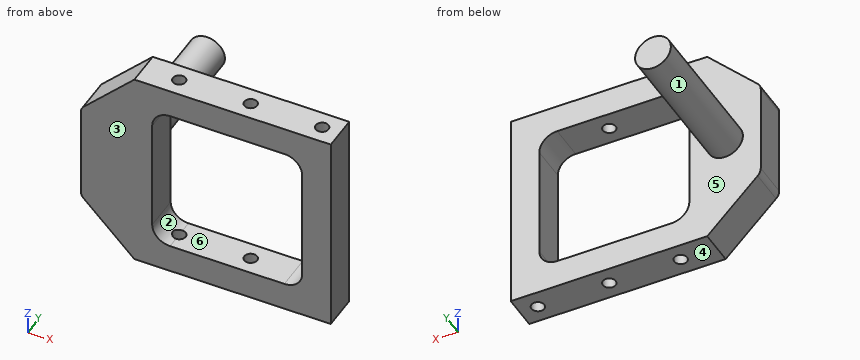
from build123d import *

# Parameters (mm, degrees)
SKETCH1_W          = 70
SKETCH1_H          = 10
EXTRUDE1_DEPTH     = 58
SKETCH2_R          = 5
EXTRUDE2_DEPTH     = 49
CUT_EXTRUDE1_DEPTH = 30
CHAMFER1_SIZE      = 15
FILLET1_R          = 3
SKETCH4_R          = 1.8
CUT_EXTRUDE2_DEPTH = 60


with BuildPart() as part:
    # Sketch1 → Extrude1 (new body)
    with BuildSketch(Plane.XY):
        with Locations((-10.032216865, -100)):
            Rectangle(SKETCH1_W, SKETCH1_H)
    extrude(amount=EXTRUDE1_DEPTH)

    # Sketch2 → Extrude2 (add)
    with BuildSketch(Plane.XZ.offset(105)):
        with Locations((-35.032216865, 28.7)):
            Circle(SKETCH2_R)
    extrude(amount=-EXTRUDE2_DEPTH)

    # Sketch3 → Cut-Extrude1 (cut)
    with BuildSketch(Plane.XZ.offset(105)):
        with BuildLine():
            Line((-20.032216865, 50), (11.967783135, 50))
            ThreePointArc((11.967783135, 50), (15.503317041, 48.535533906), (16.967783135, 45))
            Line((16.967783135, 45), (16.967783135, 13))
            ThreePointArc((16.967783135, 13), (15.503317041, 9.464466094), (11.967783135, 8))
            Line((11.967783135, 8), (-20.032216865, 8))
            ThreePointArc((-20.032216865, 8), (-23.567750771, 9.464466094), (-25.032216865, 13))
            Line((-25.032216865, 13), (-25.032216865, 45))
            ThreePointArc((-25.032216865, 45), (-23.567750771, 48.535533906), (-20.032216865, 50))
        make_face()
    extrude(amount=-CUT_EXTRUDE1_DEPTH, mode=Mode.SUBTRACT)

    # Chamfer1
    chamfer1_edges = [part.edges().sort_by_distance(p)[0] for p in [
        (-45.032216865, -100, 58),
        (-45.032216865, -100, 0),
    ]]
    chamfer(chamfer1_edges, length=CHAMFER1_SIZE)

    # Fillet1
    fillet1_edges = [part.edges().sort_by_distance(p)[0] for p in [
        (-45.032216865, -100, 43),
        (-45.032216865, -100, 15),
    ]]
    fillet(fillet1_edges, radius=FILLET1_R)

    # Sketch4 → Cut-Extrude2 (cut)
    with BuildSketch(Plane.XY.offset(58)):
        with Locations((-20.032216865, -100)):
            Circle(SKETCH4_R)
        with Locations((-0.032216865, -100)):
            Circle(SKETCH4_R)
        with Locations((19.967783135, -100)):
            Circle(SKETCH4_R)
    extrude(amount=-CUT_EXTRUDE2_DEPTH, mode=Mode.SUBTRACT)


solid = part.part
Source: CAD feature listing. Evaluate the final solid. Frame: model axes, mm. Face numbers are marked on the shaded views. A direction names the side the tool comes from. Coordinates: 2 decimals unless noted, no trailing zeros. Write each loop counter-clockwise with the first axis right and the second up, starting at its lowest first coordinate (ties: lowest second). Pieces come first, ordered by that corner, then holes. Notation, with made-up numbers: M 85,-0.5 L 97,-0.5 A28 cw 97,25.5 Z; hole C -25.5,-1.75 d9. An arc over 180 degrees is marked long. Use a Markdown table: item, result.
1) Section B-B, the plane y = -100. Give the number of separate pieces and of enclosed holes in the cut face, then the cut area to 3 significant figures.
Conclusion:
| item | result |
|---|---|
| separate pieces | 5 |
| enclosed holes | 0 |
| area | 1,770 mm^2 |
2) First-contact query: pin 1 Ø2 at (x, y) = (-0.03, -100) entering from +Z; pin 2 Ø17.5 at (x, z) = (-17, 40) entering from +Y. Flat tips, straight axial feed; report the tip coordinate or a pass-through.
Conclusion:
| item | result |
|---|---|
| pin 1 | passes through |
| pin 2 | stops at y = -95 |
3) Mould query, pull axis Z, two halves, no side actions, for the marked faces 4, 5 and 6. Classes: pulls with the +Z half, pulls with the -Z half, needs draft (parallel to the pull), parting line crosses it, or undercut.
Conclusion:
| item | result |
|---|---|
| face 4 | pulls with the -Z half |
| face 5 | needs draft |
| face 6 | undercut |
4) Section D-D, the plane x = -28. Output: boundary loops of the cut face in (y, z).
Conclusion:
| item | result |
|---|---|
| outline | M -105,0 L -95,0 L -95,58 L -105,58 Z |
5) Ray query, L1, parallel to X at y = -100, z = 28.5; L2, parallel to X at y = -96, z = 28.5; L3, parallel to Y at x = 20, z = 6.5. Return the intervals inside material, ascending.
Conclusion:
| item | result |
|---|---|
| L1 | x = -45.03 to -25.03, 16.97 to 18.17, 21.77 to 24.97 |
| L2 | x = -45.03 to -25.03, 16.97 to 24.97 |
| L3 | y = -105 to -101.8, -98.2 to -95 |
6) Reachability of the marked faces 1, 2 and 3 from +Z, -Z, +X, -X, +Y, -Y: full face, straight path, thin tool, end or side. Return the list, or none.
Conclusion:
| item | result |
|---|---|
| face 1 | +Y |
| face 2 | +Y, -Y |
| face 3 | +Z, -Z, +X, -X, -Y |
7) Section C-C, the plane z = 51.5. Output: boundary loops of the cut face in (x, y), then the cut area to 3 significant figures.
Conclusion:
| item | result |
|---|---|
| outline | M -36.53,-105 L 24.97,-105 L 24.97,-95 L -36.53,-95 Z; hole C -20.03,-100 d3.6; hole C -0.03,-100 d3.6; hole C 19.97,-100 d3.6 |
| area | 584 mm^2 |
8) Section A-A, the plane z = 28.7. Output: boundary loops of the cut face in (x, y), then the cut area to 3 significant figures.
Conclusion:
| item | result |
|---|---|
| outline | M -45.03,-105 L -25.03,-105 L -25.03,-95 L -30.03,-95 L -30.03,-56 L -40.03,-56 L -40.03,-95 L -45.03,-95 Z; M 16.97,-105 L 24.97,-105 L 24.97,-95 L 16.97,-95 Z; hole C 19.97,-100 d3.6 |
| area | 660 mm^2 |
